The listing builds one solid part. Answer for the finished solid, in the listing's coordinates (mm). Round coordinates to 2 decimals unless told otherwise and drop trailing zeros. Write each loop counter-clockwise with the first axis right and the second up, starting at its lowest first coordinate (ties: lowest second). Pieces come first, ordered by that corner, then holes. Notation, with made-up numbers: M -25.75,-12.5 L 32.25,-12.5 A22 cw 32.25,21.5 Z; hole C 76.25,73.5 d9. An arc over 180 degrees is marked long. One line per item, written item: value. Start each with the question number.
(1) Section C-C (x = -17.5) is taken. Determine the outline of the cut face in (y, z), plus the area to 3 significant figures.
(2) Section A-A (y = 5) is taken. Determine the outline of the cut face in (x, z), plus the area to 3 significant figures.
(3) Section B-B (z = -5) is taken. Determine the outline of the cut face in (x, y).
(4) Consider probe 1 along X at (y, z) = (5, -5.25); probe 2 along X at (y, z) = (5, -6.75); probe 3 along Y at (x, z) = (-142.5, -5.5). Determine where each line is inside the solid, lowest interval first.
(5) Given P1, Ø4, axis at y = 5.5, z = -6.5, coming from the +X side, flat-ended and moving along its own axis, determine where the tip first touches the part or whether it passes through.
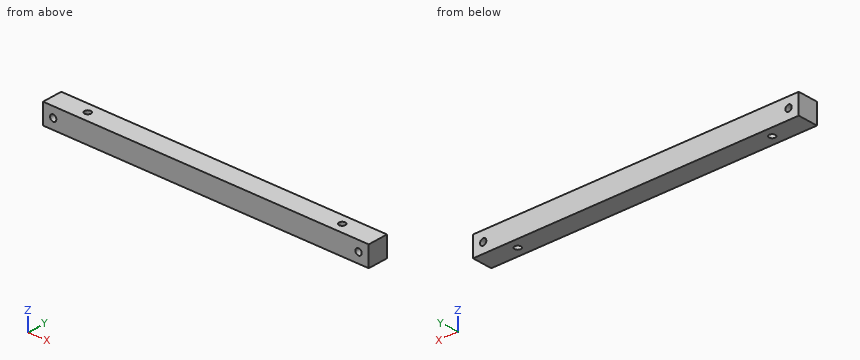
Autodesk Inventor part; units mm, degrees
ref_plane "YZ Plane" through (0, 0, 0) normal (1, 0, 0) x (0, 1, 0)
ref_plane "XZ Plane" through (0, 0, 0) normal (0, 1, 0) x (-1, 0, 0)
ref_plane "XY Plane" through (0, 0, 0) normal (0, 0, 1) x (1, 0, 0)
sketch "スケッチ1" plane through (0, 0, 0) normal (0, 1, 0) x (-1, 0, 0)
  line L0 (0, 0) -> (160, 0)
  line L1 (160, 0) -> (160, -10)
  line L2 (160, -10) -> (0, -10)
  line L3 (0, -10) -> (0, 0)
  dimension "d0" = 160
  dimension "d1" = 10
extrude "押し出し1" add sketch "スケッチ1" along normal blind 10
sketch "スケッチ2" plane through (0, 10, 0) normal (0, 1, 0) x (1, 0, 0)
  line L0 (-160, 10) -> (-160, 0)
  line L1 (0, 0) -> (0, 10)
  point P0 (-5, 5)
  point P1 (-155, 5)
  point P2 (-160, 5)
  point P3 (0, 5)
  point P4 (0, 5)
  point P5 (-160, 5)
  dimension "d4" = 5
  dimension "d5" = 5
hole "穴1" at (-5, 10, -5) at (-155, 10, -5) direction (0, -1, 0) diameter 3.1 end through all
sketch "スケッチ3" plane through (-160, 0, 0) normal (0, 0, 1) x (1, 0, 0)
  line L0 (160, 0) -> (160, 10)
  line L1 (0, 0) -> (0, 10)
  point P0 (17.5, 5)
  point P1 (142.5, 5)
  point P2 (160, 5)
  point P3 (0, 5)
  point P4 (160, 5)
  point P5 (0, 5)
  dimension "d13" = 17.5
  dimension "d14" = 17.5
hole "穴2" at (-142.5, 5, 0) at (-17.5, 5, 0) direction (0, 0, -1) diameter 3.1 end through all
properties part number "Shita"
Recorded:
1. outline: M 0,-10 L 3.45,-10 L 3.45,0 L 0,0 Z; M 6.55,-10 L 10,-10 L 10,0 L 6.55,0 Z
1. area: 69.0 mm2
2. outline: M -160,-10 L -144.05,-10 L -144.05,0 L -160,0 Z; M -140.95,-10 L -19.05,-10 L -19.05,0 L -140.95,0 Z; M -15.95,-10 L 0,-10 L 0,0 L -15.95,0 Z; hole C -155,-5 d3.1; hole C -5,-5 d3.1
2. area: 1,520 mm2
3. outline: M -160,0 L -156.55,0 L -156.55,10 L -160,10 Z; M -153.45,0 L -6.55,0 L -6.55,10 L -153.45,10 Z; M -3.45,0 L 0,0 L 0,10 L -3.45,10 Z; hole C -142.5,5 d3.1; hole C -17.5,5 d3.1
4. probe 1: x = -160 to -156.53, -153.47 to -144.05, -140.95 to -19.05, -15.95 to -6.53, -3.47 to 0
4. probe 2: x = -160 to -144.05, -140.95 to -19.05, -15.95 to 0
4. probe 3: y = 0 to 3.45, 6.55 to 10
5. P1: stops at x = 0
